Could you check a few things on this model? Use its own coordinates, in mm. A direction names the side the tool comes from. Coordinates: 2 decimals unless noted, no trailing zeros. Loops run counter-clockwise (first coordinate to the right, second up) from the corner with the lowest first, then second, coordinate; pieces in that order, holes last. Notation, with made-up numbers: (43, 42) -> (98, 42) arc R17 ccw to (98, 62) -> close; hole circle Ø6 at (-14, -30). An arc over 180 degrees is marked (long way). One line per question, with ' | ' between items.
```python
from build123d import *

# Parameters (mm, degrees)
F3_DEPTH = 12.5
F1_DEPTH = 25
F4_SIZE2 = 15
F4_SIZE  = 5
F5_SIZE  = 3
F6_R     = 2


with BuildPart() as f3:
    # F2 (on Right) → F3 (new body, symmetric)
    with BuildSketch(Plane.YZ):
        Polygon((0, 15), (0, 0), (6.5, 0), (6.5, -3), (3, -3), (3, -4.5), (8, -4.5), (8, 15), align=None)
    extrude(amount=F3_DEPTH, both=True)

    # F0 (on face) → F1 (cut)
    with BuildSketch(Plane.XY.offset(15)):
        Polygon((7.5, 8), (12.5, 4), (12.5, 8), align=None)
        Polygon((-12.5, 4), (-7.5, 8), (-12.5, 8), align=None)
    extrude(amount=-F1_DEPTH, mode=Mode.SUBTRACT)

    # F4
    f4_edges = [f3.edges().sort_by_distance(p)[0] for p in [
        (0, 8, 15),
    ]]
    chamfer(f4_edges, length=F4_SIZE, length2=F4_SIZE2)

    # F5
    f5_edges = [f3.edges().sort_by_distance(p)[0] for p in [
        (-12.5, 1.5, 15),
        (12.5, 1.5, 15),
    ]]
    chamfer(f5_edges, length=F5_SIZE)

    # F6
    f6_edges = [f3.edges().sort_by_distance(p)[0] for p in [
        (0, 8, -4.5),
    ]]
    fillet(f6_edges, radius=F6_R)


solid = f3.part
```
Q1. We'd pull the mould along Z, two halves only. Please class faces 1 (the face through (0, 4, -4.5)), 2 (the face through (0, 3, 0)), 3 (the face through (-12.5, 3.5, -3.7)): released by +Z, released by -Z, zero draft, split by the parting line, or undercut.
Values follow:
face 1: released by -Z | face 2: undercut | face 3: zero draft
Q2. For pin 1 (1.2 mm diameter, centred on x = -3.5, z = -3.5, fed in from -Y); pin 2 (1.5 mm diameter, centred on x = 0, z = -1, fed in from -Y), each with a flat end and sliding along its axis, tell me the tip position at first contact or that it passes through.
Values follow:
pin 1: stops at y = 3 | pin 2: stops at y = 6.5
Q3. Imagine slicing it at C-C on x = 8. Write out the boundary of the cut face in (y, z), plus the area to 3 significant figures.
Values follow:
outline: (0, 0) -> (6.5, 0) -> (6.5, -3) -> (3, -3) -> (3, -4.5) -> (6, -4.5) arc R2 ccw to (7.6, -3.7) -> (7.6, 1.2) -> (3, 15) -> (0, 15) -> close | area: 92.1 mm2
Q4. Please list where these lines run through material, in increasing order: L1, parallel to Z at x = 9.25, y = 0.5; L2, parallel to Y at x = 6.75, z = 0.75; L3, parallel to Y at x = 6, z = 5.5. Write a range as [from, to].
Values follow:
L1: z = [0, 15] | L2: y = [0, 7.75] | L3: y = [0, 6.17]
Q5. Imagine slicing it at D-D on z = 3. Write out the boundary of the cut face in (x, y), plus the area to 3 significant figures.
Values follow:
outline: (-12.5, 0) -> (12.5, 0) -> (12.5, 4) -> (8.75, 7) -> (-8.75, 7) -> (-12.5, 4) -> close | area: 164 mm2
Q6. For faces 4 (the face through (0, 3, -4)), 5 (the face through (0, 5, -3)), 6 (the face through (0, 8, -1)), which set-ups out of +Z, -Z, +X, -X, +Y, -Y let a thin tool reach every point of the face, with its end or its side?
Values follow:
face 4: -Z, +X, -X, -Y | face 5: +X, -X, -Y | face 6: +Z, -Z, +X, -X, +Y
Q7. Imagine slicing it at B-B on y = 0.75. Write out the boundary of the cut face in (x, z).
Values follow:
outline: (-12.5, 0) -> (12.5, 0) -> (12.5, 12) -> (9.5, 15) -> (-9.5, 15) -> (-12.5, 12) -> close
Q8. Imagine slicing it at A-A on y = 3.5. Write out the boundary of the cut face in (x, z).
Values follow:
outline: (-12.5, -4.5) -> (12.5, -4.5) -> (12.5, -3) -> (-12.5, -3) -> close; (-12.5, 0) -> (12.5, 0) -> (12.5, 12) -> (11, 13.5) -> (-11, 13.5) -> (-12.5, 12) -> close
